Autodesk Inventor part; units mm, degrees
ref_plane "Work Plane1" through (29, 0, 0) normal (0, -1, 0) x (1, 0, 0)
ref_plane "YZ Plane" through (0, 0, 0) normal (1, 0, 0) x (0, 1, 0)
ref_plane "XZ Plane" through (0, 0, 0) normal (0, 1, 0) x (-1, 0, 0)
sketch "Sketch1" plane through (0, 0, 0) normal (0, 0, 1) x (1, 0, 0)
  line L0 (-2.6667, 0) -> (25, 0)
  line L1 (25, 0) -> (25, 6)
  line L2 (25, 6) -> (4.375, 6)
  line L3 (4.375, 6) -> (3.3014, 6)
  line L4 (3.3014, 6) -> (0, 6)
  line L5 (0, 6) -> (0, 9)
  line L6 (0, 9) -> (-12, 9)
  line L7 (-12, 9) -> (-12, 5.7735)
  line L8 (-12, 5.7735) -> (-6, 5.7735)
  line L9 (-6, 5.7735) -> (-2.6667, 0)
  line L10 (-19.4, 0) -> (32.4, 0)
  line L11 (0, -1.8) -> (0, 10.8)
  line L12 (4.375, 6) -> (0, 6) construction
  dimension "d1" = 20.625
  dimension "d2" = 1.0736
  dimension "d3" = 12
  dimension "d4" = 6
  dimension "d5" = 60
  dimension "d6" = 12
  dimension "d7" = 12
  dimension "d8" = 11.547
  dimension "d9" = 18
  dimension "d26" = 25
revolve "Body" add sketch "Sketch1" angle 360 about axis through (-2.6667, 0, 0) along (1, 0, 0)
sketch "Sketch2" plane through (-12, 0, 0) normal (-1, 0, 0) x (0, 0, 1)
  circle A0 centre (0, 0) radius 5.7735
  line L0 (0, -12.6) -> (0, 12.6)
  line L1 (-12.6, 0) -> (12.6, 0)
  line L2 (5.7735, 0) -> (2.8868, -5)
  line L3 (2.8868, -5) -> (-2.8868, -5)
  line L4 (-2.8868, -5) -> (-5.7735, 0)
  line L5 (-5.7735, 0) -> (-2.8868, 5)
  line L6 (-2.8868, 5) -> (2.8868, 5)
  line L7 (2.8868, 5) -> (5.7735, 0)
extrude "Slot" add sketch "Sketch2" against normal up to next contours L7 A0 | A0 L2 | L6 L0 A0 | A0 L0 L3 | L0 L6 A0 | A0 L3 L0 | L4 A0 | A0 L5
fillet "Fillet1" radius 1.2 1 edges at (-12, -9, 0)
thread "Thread"
chamfer "Chamfer1" distance 1.0735 distance2 1.0735 1 edges at (25, -6, 0) measured on face at (25, -3.0269, -1.5886)
ref_plane "Work Plane1" through (29, 0, 0) normal (0, -1, 0) x (1, 0, 0)
fillet "Fillet2" radius 0.1 1 edges at (0, -6, 0)
equation "\"d1\" = GEL"
equation "\"d3\" = KOH"
equation "\"d4\" = INTI"
equation "\"d6\" = GD"
equation "\"d7\" = BDM"
equation "\"d8\" = 1.1547 * SW"
equation "\"d9\" = KOD"
equation "\"d26\" = NLG"
equation "\"d30\" = R"
equation "\"d17\" = RR"
equation "\"d13\" = GEL"
equation "\"d15\" = -0.5 * SPD + 0.5 * GD"
equation "\"d16\" = GUL"
equation "\"GD\" = NND"
equation "\"NLG\" = 25"
equation "\"GEL\" = 20.625"
equation "\"KOD\" = 18"
equation "\"KOH\" = NND"
equation "\"INTI\" = 6"
equation "\"GAL\" = 0.61345 * PTC"
equation "\"GUL\" = 0.61345 * PTC"
equation "\"BDM\" = NND"
equation "\"RR\" = 0.1 * NND"
equation "\"SPD\" = NND - 1.2269 * PTC"
equation "\"R\" = 0.1"
equation "\"PHH\" = 0.25"
equation "\"GD1\" = THREADDIA - 1.2269 * PTC"
equation "\"THREADDIA\" = 12"
equation "\"FAWI\" = 45deg"
equation "\"PTC\" = 1.75"
equation "\"KOH1\" = 10.8"
equation "\"NND\" = 12"
equation "\"TOA\" = 30deg"
equation "\"E0\" = 1.155 * SW"
properties part number "AS 1420 - 1973 - M12 x 25" material "Steel, Mild"
Could you check a few things on this model? Use its own coordinates, in mm. A direction names the side the tool comes from. Give positions to 0.01 mm unless a question says otherwise; leave off trailing zeros. Order: outer loops, then holes, each group sorted by start corner. A loop starts at its lowest first (then second) coordinate and runs counter-clockwise, first axis right, second up. Notation, with made-up numbers: (34.25, 74) - (90.25, 74) arc R25 cw to (90.25, 111) - close; hole circle Ø5 at (63, 71). An arc over 180 degrees is marked (long way). Return JSON: item names as keys, results as strings. Group by question number.
Q1. Will these pins go through, and if not, where does the flat tip stop? pin 1 Ø1.5 at (x, y) = (9, -2) entering from +Z; pin 2 Ø6 at (x, z) = (5.5, -4) entering from +Y; pin 3 Ø3 at (x, z) = (4, -4.5) entering from -Y.
Q2. Which directions (+Z, -Z, +X, -X, +Y, -Y) give clear straight access to the entire face, cutting with the end or side of a thin tool? Please do faces 4 (the face through (-12, -2, 5)), 5 (the face through (-9, -5, 0)).
Q3. Suppose I cut it at A-A, the plane x = 1.5. Please give me the cut outline in (y, z), and give its area (3 significant figures).
Q4. Thinking about a two-plate mould opening in Y: for faces 1 (the face through (-8.822, -2.535, -4.31)), 2 (the face through (12, -6, 0)), 3 (the face through (0, 2, -6)), which applies, pulls with the +Y half, pulls with the -Y half, needs draft (parallel to the pull), parting line crosses it, or undercut?
Q5. Please list where these lines run through material, in increasing order: line 1 along Z through (x, y) = (-2.5, 0); line 2 along Z through (x, y) = (-5, -0.75); line 3 along Y through (x, z) = (-8.5, 1.25). Write a range as [from, to].
Resolved:
{
 "1": {"pin 1": "stops at z = 5.87", "pin 2": "stops at y = 5.92", "pin 3": "stops at y = -5.2"},
 "2": {"face 4": "+Z, -Z, -X, +Y, -Y", "face 5": "-X"},
 "3": {"outline": "circle Ø12 at (0, 0)", "area": "113 mm2"},
 "4": {"face 1": "undercut", "face 2": "parting line crosses it", "face 3": "needs draft"},
 "5": {"line 1": "z = [-9, 9]", "line 2": "z = [-8.97, -3.97], [3.97, 8.97]", "line 3": "y = [-8.91, -5], [5, 8.91]"}
}
